The model under review builds one solid part; all positions refer to its coordinate system, in mm. A direction names the side the tool comes from. Round coordinates to 2 decimals unless told otherwise and drop trailing zeros.
1) Mouldability with a two-part tool opening along Z and no side actions: class faces 1 (the face through (-12, -43, -0.905)), 2 (the face through (54, 8, -13.705)), 3 (the face through (53, -7, -20.105)), 4 (the face through (-18.518, -44.284, -5.316)) as pulls with the +Z half, pulls with the -Z half, needs draft (parallel to the pull), parting line crosses it, or undercut.
2) Clearance check with flat-ended pins moving along their axes: P1, Ø5, axis at y = -9.5, z = -17.5, coming from the +X side; P2, Ø2.5, axis at x = -52.5, z = -16, coming from the +Y side; P3, Ø3, axis at x = -18.5, z = -7.5, coming from the -Y side; P4, Ø4, axis at x = -26.5, y = -30, coming from the -Z side. State where each tip first meets the part, or that it passes through.
3) To check wall thickness, follow L1, parallel to Y at x = 0, z = -2.8; L2, parallel to X at y = 1.5, z = -6.5; L3, parallel to X at y = 26, z = -5. State the ranges of each line that lie inside material, in increasing order.
4) Machinability: for faces 5 (the face through (55.4, 0.3, -9.9)), 6 (the face through (-55.4, -0.3, -9.9)), 7 (the face through (18.518, 44.284, -5.316)), 8 (the face through (54, 4, -18.585)), 9 (the face through (-24, -42, -4.505)), which of the approach directions +Z, -Z, +X, -X, +Y, -Y give a long, thin tool a straight path to every point of the face, cutting with its end or side? Answer none if there is none.
from build123d import *
from build123d.topology import SkipClean

# Parameters (mm, degrees)
CROQUIS1_R              = 75
SALIENTE_EXTRUIR1_DEPTH = 6.5
CROQUIS2_R              = 69.25
CROQUIS2_R_2            = 66.5
SALIENTE_EXTRUIR2_DEPTH = 17.5
REDONDEO1_R             = 10
CROQUIS5_R              = 60
CORTAR_EXTRUIR2_DEPTH   = 121.5
CORTAR_EXTRUIR3_START   = 121.5
CROQUIS6_R              = 66.5
CORTAR_EXTRUIR3_DEPTH   = 121.5
CORTAR_EXTRUIR4_START   = -2
CROQUIS7_R              = 63
CROQUIS7_R_2            = 60
CORTAR_EXTRUIR4_DEPTH   = 1.5
CORTAR_EXTRUIR5_DEPTH   = 3.5
CROQUIS9_R              = 65.632503002
CROQUIS9_R_2            = 55
SALIENTE_EXTRUIR3_DEPTH = 3
CORTAR_EXTRUIR7_DEPTH   = 90
MATRIZC1_COUNT          = 2
CROQUIS11_OUTSIDE_W     = 194.698
CROQUIS11_OUTSIDE_H     = 194.698
CROQUIS11_OUTSIDE_R     = 71.5
CORTAR_EXTRUIR8_DEPTH   = 61
ESCALA1_SCALE           = 0.8


with BuildPart() as part:
    # Croquis1 → Saliente-Extruir1 (new body)
    with BuildSketch(Plane.XY):
        Circle(CROQUIS1_R)
    extrude(amount=-SALIENTE_EXTRUIR1_DEPTH)

    # Croquis2 → Saliente-Extruir2 (add)
    with BuildSketch(Plane(origin=(0, 0, -6.5), x_dir=(-1, 0, 0), z_dir=(0, 0, -1))):
        with Locations(Location((0, 0, 0), (0, 0, 180))):
            Circle(CROQUIS2_R)
        Circle(CROQUIS2_R_2, mode=Mode.SUBTRACT)
    extrude(amount=SALIENTE_EXTRUIR2_DEPTH)

    # Redondeo1
    # the kernel refuses this fillet: 10 mm, written as the material it takes off along each edge
    with BuildSketch(Plane(origin=(0, 0, 0), x_dir=(1, 0, 0), z_dir=(0, -1, 0))) as redondeo1_piece_1:
        with BuildLine():
            CenterArc((65.632503002, -10), REDONDEO1_R, 20.487315115, 69.512684885)
            Line((65.632503002, 0), (65.632503002, 0.2))
            Line((65.632503002, 0.2), (75, 0.2))
            Line((75, 0.2), (75.2, 0))
            ThreePointArc((75.2, 0), (75.2, -3.25), (75.18734994, -6.43))
            Line((75.18734994, -6.43), (75, -6.5))
        make_face()
    revolve(axis=Axis((0, 0, 0), (0, 0, 1)), mode=Mode.SUBTRACT)

    # Croquis5 → Cortar-Extruir2 (cut)
    with BuildSketch(Plane(origin=(0, 0, -6.5), x_dir=(-1, 0, 0), z_dir=(0, 0, -1))):
        Circle(CROQUIS5_R)
    extrude(amount=-CORTAR_EXTRUIR2_DEPTH, mode=Mode.SUBTRACT)

    # Croquis6 → Cortar-Extruir3 (cut)
    with BuildSketch(Plane(origin=(0, 0, -6.5), x_dir=(-1, 0, 0), z_dir=(0, 0, -1)).offset(CORTAR_EXTRUIR3_START)):
        with BuildLine():
            ThreePointArc((53.795389167, 0), (-11.643453263, -52.520223645), (-48.755180109, 22.734913859))
            Line((-48.755180109, 22.734913859), (-54.378467222, 25.357095704))
            ThreePointArc((-54.378467222, 25.357095704), (-12.986376836, -58.577760427), (60, 0))
            ThreePointArc((60, 0), (58.577760427, 12.986376836), (54.378467222, 25.357095704))
            Line((54.378467222, 25.357095704), (48.755180109, 22.734913859))
            ThreePointArc((48.755180109, 22.734913859), (52.520223645, 11.643453263), (53.795389167, 0))
        make_face()
        with BuildLine():
            Line((-54.378467222, 25.357095704), (-48.755180109, 22.734913859))
            ThreePointArc((-48.755180109, 22.734913859), (0, 53.795389167), (48.755180109, 22.734913859))
            Line((48.755180109, 22.734913859), (54.378467222, 25.357095704))
            ThreePointArc((54.378467222, 25.357095704), (0, 60), (-54.378467222, 25.357095704))
        make_face()
        Circle(CROQUIS6_R)
        with BuildLine():
            Line((0, 0), (76.100368106, 35.486184436))
            ThreePointArc((76.100368106, 35.486184436), (0, 83.967465793), (-76.100368106, 35.486184436))
            Line((-76.100368106, 35.486184436), (0, 0))
        make_face()
        with BuildLine():
            ThreePointArc((60, 0), (-12.986376836, -58.577760427), (-54.378467222, 25.357095704))
            Line((-54.378467222, 25.357095704), (-60.269467838, 28.104114406))
            ThreePointArc((-60.269467838, 28.104114406), (-14.393234327, -64.923684473), (66.5, 0))
            ThreePointArc((66.5, 0), (64.923684473, 14.393234327), (60.269467838, 28.104114406))
            Line((60.269467838, 28.104114406), (54.378467222, 25.357095704))
            ThreePointArc((54.378467222, 25.357095704), (58.577760427, 12.986376836), (60, 0))
        make_face()
        with BuildLine():
            Line((-60.269467838, 28.104114406), (-54.378467222, 25.357095704))
            ThreePointArc((-54.378467222, 25.357095704), (0, 60), (54.378467222, 25.357095704))
            Line((54.378467222, 25.357095704), (60.269467838, 28.104114406))
            ThreePointArc((60.269467838, 28.104114406), (0, 66.5), (-60.269467838, 28.104114406))
        make_face()
    cortar_extruir3 = extrude(amount=-CORTAR_EXTRUIR3_DEPTH, mode=Mode.SUBTRACT)

    # Croquis7 → Cortar-Extruir4 (cut)
    with BuildSketch(Plane(origin=(0, 0, -6.5), x_dir=(-1, 0, 0), z_dir=(0, 0, -1)).offset(CORTAR_EXTRUIR4_START)):
        Circle(CROQUIS7_R)
        Circle(CROQUIS7_R_2, mode=Mode.SUBTRACT)
    extrude(amount=-CORTAR_EXTRUIR4_DEPTH, mode=Mode.SUBTRACT)

    # Croquis8 → Cortar-Extruir5 (cut)
    with SkipClean():  # the faces are left unmerged after this step: merging them gives an invalid solid
        with BuildSketch(Plane(origin=(0, 0, -6.5), x_dir=(-1, 0, 0), z_dir=(0, 0, -1))):
            with BuildLine():
                Line((59.77659711, 19.893678341), (-54.920166384, -30.867058887))
                ThreePointArc((-54.920166384, -30.867058887), (-57.610247866, -25.49626131), (-59.77659711, -19.893678341))
                Line((-59.77659711, -19.893678341), (54.920166384, 30.867058887))
                ThreePointArc((54.920166384, 30.867058887), (57.610247866, 25.49626131), (59.77659711, 19.893678341))
            make_face()
        extrude(amount=-CORTAR_EXTRUIR5_DEPTH, mode=Mode.SUBTRACT)

    # Croquis9 → Saliente-Extruir3 (add)
    with SkipClean():  # the faces are left unmerged after this step: merging them gives an invalid solid
        with BuildSketch(Plane.XY):
            Circle(CROQUIS9_R)
            Circle(CROQUIS9_R_2, mode=Mode.SUBTRACT)
        extrude(amount=-SALIENTE_EXTRUIR3_DEPTH)

    # Simetría1: Cortar-Extruir3 across plane
    with SkipClean():  # the faces are left unmerged after this step: merging them gives an invalid solid
        add(cortar_extruir3.mirror(Plane.ZX), mode=Mode.SUBTRACT)

    # Croquis10 → Cortar-Extruir7 (cut)
    with SkipClean():  # the faces are left unmerged after this step: merging them gives an invalid solid
        with BuildSketch(Plane(origin=(0, 0, 0), x_dir=(0, 0, -1), z_dir=(1, 0, 0))):
            with BuildLine():
                Line((20.1, -17.78519151), (24, -17.78519151))
                Line((24, -17.78519151), (24, -11.68519151))
                Line((24, -11.68519151), (22.6, -11.68519151))
                ThreePointArc((22.6, -11.68519151), (22.246446609, -11.538744901), (22.1, -11.18519151))
                Line((22.1, -11.18519151), (22.1, -3.05))
                Line((22.1, -3.05), (22.1, 2.55))
                ThreePointArc((22.1, 2.55), (21.953553391, 2.903553391), (21.6, 3.05))
                Line((21.6, 3.05), (11.95, 3.05))
                ThreePointArc((11.95, 3.05), (11.596446609, 2.903553391), (11.45, 2.55))
                Line((11.45, 2.55), (11.45, -2.55))
                ThreePointArc((11.45, -2.55), (11.596446609, -2.903553391), (11.95, -3.05))
                Line((11.95, -3.05), (15.5, -3.05))
                ThreePointArc((15.5, -3.05), (15.853553391, -3.196446609), (16, -3.55))
                Line((16, -3.55), (16, -11.68519151))
                Line((16, -11.68519151), (16, -17.28519151))
                ThreePointArc((16, -17.28519151), (16.146446609, -17.638744901), (16.5, -17.78519151))
                Line((16.5, -17.78519151), (20.1, -17.78519151))
            make_face()
        cortar_extruir7 = extrude(amount=-CORTAR_EXTRUIR7_DEPTH, mode=Mode.SUBTRACT)

    # MatrizC1: Cortar-Extruir7 ×2 about axis
    with SkipClean():  # the faces are left unmerged after this step: merging them gives an invalid solid
        matrizc1_axis = Axis((0, 0, 0), (0, 0, 1))
        for i in range(1, MATRIZC1_COUNT):
            add(cortar_extruir7.rotate(matrizc1_axis, i * 360 / MATRIZC1_COUNT), mode=Mode.SUBTRACT)

    # Croquis11 outside → Cortar-Extruir8 (cut)
    with SkipClean():  # the faces are left unmerged after this step: merging them gives an invalid solid
        with BuildSketch(Plane(origin=(0, 0, -6.5), x_dir=(-1, 0, 0), z_dir=(0, 0, -1))):
            Rectangle(CROQUIS11_OUTSIDE_W, CROQUIS11_OUTSIDE_H)
            Circle(CROQUIS11_OUTSIDE_R, mode=Mode.SUBTRACT)
        extrude(amount=-CORTAR_EXTRUIR8_DEPTH, mode=Mode.SUBTRACT)


with BuildPart() as part_1:
    # Escala1: scaled about (1.06e-07, 2.2e-08, -4.523321709)
    add(part.part.scale(ESCALA1_SCALE).moved(Location((2.1e-08, 4e-09, -0.904664342))))


solid = part_1.part
Answer below:
1. face 1: pulls with the +Z half
1. face 2: undercut
1. face 3: pulls with the -Z half
1. face 4: needs draft
2. P1: stops at x = 54.96
2. P2: stops at y = 21.04
2. P3: stops at y = -54.31
2. P4: passes through
3. L1: y = -57.2 to -44, 44 to 57.2
3. L2: x = -55.38 to -53.18, 53.18 to 55.38
3. L3: x = -50.95 to -40.35, 40.35 to 50.95
4. face 5: -Z, +X
4. face 6: -Z, -X
4. face 7: -Z
4. face 8: +X
4. face 9: none
